Source: CAD feature listing. Evaluate the final solid. Frame: model axes, mm. A direction names the side the tool comes from. Round coordinates to 2 decimals unless told otherwise and drop trailing zeros. Write each loop counter-clockwise with the first axis right and the second up, starting at its lowest first coordinate (ties: lowest second). Pieces come first, ordered by that corner, then holes. Notation, with made-up numbers: M -22,-26 L 20,-26 A8 cw 20,-19 Z; hole C 36,-35.5 d6. An arc over 180 degrees is marked long. Answer in a Markdown table with one row per item.
from build123d import *

# Parameters (mm, degrees)
SKETCH1_W           = 25.6032
SKETCH1_H           = 36.25342
SKETCH1_R           = 5.1
BOSS_EXTRUDE1_DEPTH = 1
CUT_EXTRUDE1_DEPTH  = 50.8


with BuildPart() as part:
    # Sketch1 → Boss-Extrude1 (new body)
    with BuildSketch(Plane(origin=(0, 0, 0), x_dir=(1, 0, 0), z_dir=(0, -0.7071067811865488, 0.7071067811865464))):
        with Locations((-15.465234019, -18.12671)):
            Rectangle(SKETCH1_W, SKETCH1_H)
        with Locations(Location((-15.367622747, -27.2796, 0), (0, 0, 270))):
            Circle(SKETCH1_R, mode=Mode.SUBTRACT)
    extrude(amount=BOSS_EXTRUDE1_DEPTH)

    # Sketch2 → Cut-Extrude1 (cut)
    with BuildSketch(Plane(origin=(0, 0, 0), x_dir=(1, 0, 0), z_dir=(0, 1, 0))):
        Polygon((-2.663634019, 0), (-2.663634019, 4.06654), (-7.235634019, 4.06654), (-7.235634019, 8.76554), (-2.663634019, 8.76554), (3.686238972, 8.76554), (3.686238972, -11.022964716), (-35.05379443, -11.022964716), (-35.05379443, 8.76554), (-23.694834019, 8.76554), (-23.694834019, 4.06654), (-28.266834019, 4.06654), (-28.266834019, 0), align=None)
    extrude(amount=-CUT_EXTRUDE1_DEPTH, mode=Mode.SUBTRACT)


solid = part.part
Q1. Section A-A (x = -13.5). Return loops of the section in (y, z).
Solutions:
| item | result |
|---|---|
| outline | M -26.34,-24.93 L -25.64,-25.64 L -22.65,-22.65 L -23.35,-21.94 Z; M -16.64,-15.23 L -15.93,-15.93 L 0,0 L -1.41,0 Z |
Q2. Section C-C (z = -8). Return loops of the section in (x, y), and give its area (3 significant figures).
Solutions:
| item | result |
|---|---|
| outline | M -23.69,-9.41 L -7.24,-9.41 L -7.24,-8 L -23.69,-8 Z |
| area | 23.3 mm2 |
Q3. Access query for faces 1 (the flat face through (-26, -5, -4.067)), 2 (the flat face through (-26, -9, -8.766)), 3 (the flat face through (-7.236, -7, -6)). Directions: +Z, -Z, +X, -X, +Y, -Y. A direction counts if a zero-diameter tool reaches every point of the face in a straight line with its end or side. Return the directions, or none.
Solutions:
| item | result |
|---|---|
| face 1 | -Z, -X, +Y, -Y |
| face 2 | +Z, -X, +Y, -Y |
| face 3 | +X, +Y, -Y |
Q4. Section D-D (y = -3.5). Return loops of the section in (x, z), and give its area (3 significant figures).
Solutions:
| item | result |
|---|---|
| outline | M -28.27,-3.5 L -2.66,-3.5 L -2.66,-2.09 L -28.27,-2.09 Z |
| area | 36.2 mm2 |
Q5. Pull-direction query (X, two-part tool) for faces 4 (the cylindrical face through (-20.346, -18.856, -18.159)), 5 (the flat face through (-15.644, -13.704, -12.289)), 6 (the flat face through (-28.267, -3, -2)); classes: pulls with the +X half, pulls with the -X half, needs draft (parallel to the pull), parting line crosses it, or undercut.
Solutions:
| item | result |
|---|---|
| face 4 | undercut |
| face 5 | needs draft |
| face 6 | pulls with the -X half |
Q6. Material intervals for probe 1 along Z at (x, y) = (-8, -21); probe 2 along Y at (x, z) = (-8.5, -24.5); probe 3 along Z at (x, y) = (-8, -18), sorted ascending.
Solutions:
| item | result |
|---|---|
| probe 1 | z = -21 to -19.59 |
| probe 2 | y = -25.91 to -24.5 |
| probe 3 | z = -18 to -16.59 |
Q7. Section B-B (y = -9.5). Return loops of the section in (x, z).
Solutions:
| item | result |
|---|---|
| outline | M -28.27,-9.5 L -2.66,-9.5 L -2.66,-8.77 L -7.24,-8.77 L -7.24,-8.09 L -23.69,-8.09 L -23.69,-8.77 L -28.27,-8.77 Z |
Q8. Contact query for flat-ended pins moving along their axis: pin 1 Ø4 at (y, z) = (-7.5, -5.5) entering from +X; pin 2 Ø1.4 at (y, z) = (-8.5, -5.5) entering from -X; pin 3 Ø0.7 at (x, y) = (-25.5, -10) entering from +Z; pin 4 Ø4 at (x, z) = (-25, -12.5) entering from -Y. Output: stop coordinate, or through.
Solutions:
| item | result |
|---|---|
| pin 1 | stops at x = -7.24 |
| pin 2 | passes through |
| pin 3 | stops at z = -8.77 |
| pin 4 | stops at y = -15.91 |
